```python
from build123d import *

# Parameters (mm, degrees)
SKIZZE1_R                       = 11.5
SKIZZE1_R_2                     = 8.5
AUFSATZ_LINEAR_AUSTRAGEN1_DEPTH = 4
VERRUNDUNG1_R                   = 0.5


with BuildPart() as part:
    # Skizze1 → Aufsatz-Linear austragen1 (new body)
    with BuildSketch(Plane(origin=(0, 0, 0), x_dir=(1, 0, 0), z_dir=(0, 1, 0))):
        Circle(SKIZZE1_R)
        Circle(SKIZZE1_R_2, mode=Mode.SUBTRACT)
    extrude(amount=AUFSATZ_LINEAR_AUSTRAGEN1_DEPTH)

    # Verrundung1
    verrundung1_edges = [part.edges().sort_by_distance(p)[0] for p in [
        (-11.5, 0, 0),
        (-11.5, 4, 0),
        (-8.5, 0, 0),
        (-8.5, 4, 0),
    ]]
    fillet(verrundung1_edges, radius=VERRUNDUNG1_R)


solid = part.part
```
Input: part model. Units: mm. Frame: model coordinates. Coordinates: 2 decimals unless noted, no trailing zeros. Loops run counter-clockwise (first coordinate to the right, second up) from the corner with the lowest first, then second, coordinate; pieces in that order, holes last. Notation, with made-up numbers: M 31,38 L 45,38 A9 ccw 45,55 Z; hole C 51.5,33.5 d9. An arc over 180 degrees is marked long. Answer in a Markdown table with one row per item.
1. Material intervals for line 1 (X direction, y = 1.4, z = 0); line 2 (X direction, y = 3.85, z = 2), sorted ascending.
Response:
| item | result |
|---|---|
| line 1 | x = -11.5 to -8.5, 8.5 to 11.5 |
| line 2 | x = -11.18 to -8.41, 8.41 to 11.18 |
2. First-contact query: pin 1 (1 mm diameter, centred on y = 1, z = 9, fed in from +X); pin 2 (1 mm diameter, centred on x = 7.5, y = 2.5, fed in from +Z); pin 3 (1 mm diameter, centred on y = 2, z = 2, fed in from -X). Flat tips, straight axial feed; report the tip coordinate or a pass-through.
Response:
| item | result |
|---|---|
| pin 1 | stops at x = 7.75 |
| pin 2 | stops at z = 9.12 |
| pin 3 | stops at x = -11.4 |
3. Section A-A, the plane z = 0. Output: boundary loops of the cut face in (x, y).
Response:
| item | result |
|---|---|
| outline | M -11.5,0.5 A0.5 ccw -11,0 L -9,0 A0.5 ccw -8.5,0.5 L -8.5,3.5 A0.5 ccw -9,4 L -11,4 A0.5 ccw -11.5,3.5 Z; M 8.5,0.5 A0.5 ccw 9,0 L 11,0 A0.5 ccw 11.5,0.5 L 11.5,3.5 A0.5 ccw 11,4 L 9,4 A0.5 ccw 8.5,3.5 Z |
4. Draft query along Z for faces 1 (the flat face through (2, 4, 9)), 2 (the cylindrical face through (-1.5, 2, -11.4)), 3 (the cylindrical face through (4.57, 1.979, -7.167)). Return one class per face: pulls with the +Z half, pulls with the -Z half, needs draft (parallel to the pull), parting line crosses it, or undercut.
Response:
| item | result |
|---|---|
| face 1 | needs draft |
| face 2 | parting line crosses it |
| face 3 | undercut |
5. Section C-C, the plane y = 1.95. Output: boundary loops of the cut face in (x, z).
Response:
| item | result |
|---|---|
| outline | C 0,0 d23; hole C 0,0 d17 |
6. Section B-B, the plane x = 0. Output: boundary loops of the cut face in (y, z), then the cut area to 3 significant figures.
Response:
| item | result |
|---|---|
| outline | M 0,-11 A0.5 ccw 0.5,-11.5 L 3.5,-11.5 A0.5 ccw 4,-11 L 4,-9 A0.5 ccw 3.5,-8.5 L 0.5,-8.5 A0.5 ccw 0,-9 Z; M 0,9 A0.5 ccw 0.5,8.5 L 3.5,8.5 A0.5 ccw 4,9 L 4,11 A0.5 ccw 3.5,11.5 L 0.5,11.5 A0.5 ccw 0,11 Z |
| area | 23.6 mm2 |
